from build123d import *

# Parameters (mm, degrees)
SKETCH1_W                      = 150
SKETCH1_H                      = 60
BOSS_EXTRUDE1_DEPTH            = 17.5
SKETCH2_W                      = 25.43
SKETCH2_H                      = 50.83
CUT_EXTRUDE1_DEPTH             = 50.8
CUT_EXTRUDE2_REACH             = 84.651
SKETCH3_R                      = 14.2875
CUT_EXTRUDE2_DIRECTION_2_REACH = 84.651


with BuildPart() as part:
    # Sketch1 → Boss-Extrude1 (new, symmetric)
    with BuildSketch(Plane.XY):
        Rectangle(SKETCH1_W, SKETCH1_H)
    extrude(amount=BOSS_EXTRUDE1_DEPTH, both=True)

    # Sketch2 → Cut-Extrude1 (cut)
    with BuildSketch(Plane(origin=(75, 0, 0), x_dir=(0, 0, -1), z_dir=(1, 0, 0))):
        Rectangle(SKETCH2_W, SKETCH2_H)
    cut_extrude1 = extrude(amount=-CUT_EXTRUDE1_DEPTH, mode=Mode.SUBTRACT)

    # Cut-Extrude2: up to this face of the body (flat: up to its plane)
    cut_extrude2_end = Plane(part.part.faces().sort_by_distance((0, 0, 17.5))[0])
    # Sketch3 → Cut-Extrude2 (cut, up to the picked face)
    with BuildSketch(Plane.XY, mode=Mode.PRIVATE) as cut_extrude2_sk1:
        with Locations(Location((0, 0, 0), (0, 0, 180))):
            Circle(SKETCH3_R)
    cut_extrude2_tool1 = split(extrude(cut_extrude2_sk1.sketch, amount=CUT_EXTRUDE2_REACH, mode=Mode.PRIVATE), bisect_by=cut_extrude2_end, keep=Keep.BOTH, mode=Mode.PRIVATE)
    add(cut_extrude2_tool1.solids().sort_by(Axis((0, 0, 0), (0, 0, 1)))[0], mode=Mode.SUBTRACT)

    # Cut-Extrude2 direction 2: up to this face of the body (flat: up to its plane)
    cut_extrude2_direction_2_end = Plane(part.part.faces().sort_by_distance((0, 0, -17.5))[0])
    # Sketch3 → Cut-Extrude2 direction 2 (cut, up to the picked face)
    with BuildSketch(Plane.XY, mode=Mode.PRIVATE) as cut_extrude2_direction_2_sk1:
        with Locations(Location((0, 0, 0), (0, 0, 180))):
            Circle(SKETCH3_R)
    cut_extrude2_direction_2_tool1 = split(extrude(cut_extrude2_direction_2_sk1.sketch, amount=-CUT_EXTRUDE2_DIRECTION_2_REACH, mode=Mode.PRIVATE), bisect_by=cut_extrude2_direction_2_end, keep=Keep.BOTH, mode=Mode.PRIVATE)
    add(cut_extrude2_direction_2_tool1.solids().sort_by(Axis((0, 0, 0), (0, 0, -1)))[0], mode=Mode.SUBTRACT)

    # Mirror1: Cut-Extrude1 across plane
    add(cut_extrude1.mirror(Plane(origin=(0, 0, 0), x_dir=(0, 0, 1), z_dir=(1, 0, 0))), mode=Mode.SUBTRACT)


solid = part.part
Geometry: final body of the model. Coordinates: model frame, mm. A direction names the side the tool comes from. Round coordinates to 2 decimals unless told otherwise and drop trailing zeros. Loops run counter-clockwise (first coordinate to the right, second up) from the corner with the lowest first, then second, coordinate; pieces in that order, holes last. Notation, with made-up numbers: (5.5, 47) - (63.5, 47) arc R20 ccw to (63.5, 58) - close; hole circle Ø8 at (48.25, -32). An arc over 180 degrees is marked (long way). Write each question's results on one line, items separated by ' | '. Start each with the question number.
1) Cut plane B-B on x = 33. Return loops of the section in (y, z) (3 decimals), then the cut area to 3 significant figures.
2) Mould query, pull axis Y, two halves, no side actions, for faces 1 (the face through (-75, 0, -15)), 2 (the face through (-50, 25.415, 0)), 3 (the face through (-1, -30, 0)). Classes: released by +Y, released by -Y, zero draft, split by the parting line, or undercut.
3) Line query: probe 1 along Y at (x, z) = (53, -11) (3 decimals); probe 2 along Y at (x, z) = (0, -10); probe 3 along Z at (x, y) = (54, 4) (3 decimals). Output: solid intervals per line, ascending. Write a range as [from, to].
4) Cut plane C-C on y = 19. Return loops of the section in (x, z) (3 decimals).
5) Cut plane A-A on x = 0. Return loops of the section in (y, z).
6) First-contact query: P1, Ø5, axis at y = 0, z = 9, coming from the +X side; P2, Ø10, axis at y = 5.5, z = 2.5, coming from the -X side. Flat tips, straight axial feed; report the tip coordinate or a pass-through.
7) Access query for faces 4 (the face through (-50, 0, 12.715)), 5 (the face through (50, 25.415, 0)), 6 (the face through (-1, 30, 0)). Directions: +Z, -Z, +X, -X, +Y, -Y. A direction counts if a zero-diameter tool reaches every point of the face in a straight line with its end or side. Return the directions, or none.
8) Cut plane D-D on y = 0. Return loops of the section in (x, z) (1 decimal).
Verdict:
1) outline: (-30, -17.5) - (30, -17.5) - (30, 17.5) - (-30, 17.5) - close; hole (-25.415, -12.715) - (25.415, -12.715) - (25.415, 12.715) - (-25.415, 12.715) - close | area: 807 mm2
2) face 1: zero draft | face 2: undercut | face 3: released by -Y
3) probe 1: y = [-30, -25.415], [25.415, 30] | probe 2: y = [-30, -14.29], [14.29, 30] | probe 3: z = [-17.5, -12.715], [12.715, 17.5]
4) outline: (-75, -17.5) - (75, -17.5) - (75, -12.715) - (24.2, -12.715) - (24.2, 12.715) - (75, 12.715) - (75, 17.5) - (-75, 17.5) - (-75, 12.715) - (-24.2, 12.715) - (-24.2, -12.715) - (-75, -12.715) - close
5) outline: (-30, -17.5) - (-14.29, -17.5) - (-14.29, 17.5) - (-30, 17.5) - close; (14.29, -17.5) - (30, -17.5) - (30, 17.5) - (14.29, 17.5) - close
6) P1: stops at x = 24.2 | P2: stops at x = -24.2
7) face 4: -X | face 5: +X | face 6: +Z, -Z, +X, -X, +Y
8) outline: (-75, -17.5) - (-14.3, -17.5) - (-14.3, 17.5) - (-75, 17.5) - (-75, 12.7) - (-24.2, 12.7) - (-24.2, -12.7) - (-75, -12.7) - close; (14.3, -17.5) - (75, -17.5) - (75, -12.7) - (24.2, -12.7) - (24.2, 12.7) - (75, 12.7) - (75, 17.5) - (14.3, 17.5) - close
